Read the model definition and answer for the solid it produces. Units are mm, in the model's axes. A direction names the side the tool comes from. Coordinates: 2 decimals unless noted, no trailing zeros. Loops run counter-clockwise (first coordinate to the right, second up) from the corner with the lowest first, then second, coordinate; pieces in that order, holes last. Notation, with made-up numbers: (54, -11) - (86, -11) arc R7 cw to (86, -1) - close; hole circle Ø6 at (71.25, 7.25). An arc over 180 degrees is marked (long way). Use one line per item in the form item = value.
Autodesk Inventor part; units mm, degrees
ref_plane "YZ Plane" through (0, 0, 0) normal (1, 0, 0) x (0, 1, 0)
ref_plane "XZ Plane" through (0, 0, 0) normal (0, 1, 0) x (-1, 0, 0)
ref_plane "XY Plane" through (0, 0, 0) normal (0, 0, 1) x (1, 0, 0)
sketch "Sketch1" plane through (0, 0, 0) normal (0, 1, 0) x (-1, 0, 0)
  circle A0 centre (0, 12.75) radius 8.05
  circle A1 centre (0, -12.75) radius 8.05
  line L0 (14.5, 27) -> (-14.5, 27)
  line L1 (-14.5, 27) -> (-14.5, -27)
  line L2 (-14.5, -27) -> (14.5, -27)
  line L3 (14.5, -27) -> (14.5, 27)
  line L4 (14.5, 27) -> (-14.5, -27) construction
  line L5 (-14.5, 27) -> (14.5, -27) construction
  point P0 (0, 0)
  dimension "d0" = 16.1
  dimension "d1" = 16.1
  dimension "d2" = 25.5
  dimension "d3" = 29
  dimension "d4" = 54
  dimension "d5" = 14.5
  dimension "d6" = 14.5
  dimension "d7" = 14.25
  dimension "d8" = 14.25
extrude "Extrusion1" add sketch "Sketch1" along normal blind 3
sketch "Sketch2" plane through (0, 3, 0) normal (0, 1, 0) x (1, 0, 0)
  line L0 (-11.5, -24) -> (11.5, -24)
  line L1 (11.5, -24) -> (11.5, 24)
  line L2 (11.5, 24) -> (-11.5, 24)
  line L3 (-11.5, 24) -> (-11.5, -24)
  line L4 (-11.5, -24) -> (11.5, 24) construction
  line L5 (11.5, -24) -> (-11.5, 24) construction
  line L6 (14.5, -27) -> (14.5, 27)
  line L7 (-14.5, -27) -> (14.5, -27)
  line L8 (14.5, -27) -> (14.5, 27)
  line L9 (14.5, 27) -> (-14.5, 27)
  line L10 (-14.5, 27) -> (-14.5, -27)
  line L11 (-14.5, -27) -> (14.5, 27) construction
  line L12 (14.5, -27) -> (-14.5, 27) construction
  point P0 (0, 0)
  dimension "d11" = 23
  dimension "d12" = 48
extrude "Extrusion2" add sketch "Sketch2" along normal blind 25
sketch "Sketch3" plane through (0, 28, 0) normal (0, 1, 0) x (1, 0, 0)
  line L0 (-25.5, 27) -> (25.5, 27)
  line L1 (25.5, 27) -> (25.5, -27)
  line L2 (25.5, -27) -> (-25.5, -27)
  line L3 (-25.5, -27) -> (-25.5, 27)
  line L4 (-25.5, 27) -> (25.5, -27) construction
  line L5 (25.5, 27) -> (-25.5, -27) construction
  line L6 (14.5, -27) -> (14.5, 27)
  line L7 (-14.5, 27) -> (14.5, 27)
  line L8 (14.5, 27) -> (14.5, -27)
  line L9 (14.5, -27) -> (-14.5, -27)
  line L10 (-14.5, -27) -> (-14.5, 27)
  line L11 (-14.5, 27) -> (14.5, -27) construction
  line L12 (14.5, 27) -> (-14.5, -27) construction
  point P0 (0, 0)
  dimension "d15" = 51
extrude "Extrusion3" add sketch "Sketch3" against normal blind 3 contours L0 L10 L2 L3 | L0 L1 L2 L6
sketch "Sketch4" plane through (0, 28, 0) normal (0, 1, 0) x (1, 0, 0)
  line L0 (-25.5, -27) -> (25.5, -27)
  line L1 (-25.5, 27) -> (25.5, 27)
  line L2 (25.5, 27) -> (25.5, -27)
  line L3 (25.5, -27) -> (-25.5, -27)
  line L4 (-25.5, -27) -> (-25.5, 27)
  line L5 (-25.5, 27) -> (25.5, -27) construction
  line L6 (25.5, 27) -> (-25.5, -27) construction
  line L7 (-22.5, 24) -> (22.5, 24)
  line L8 (22.5, 24) -> (22.5, -24)
  line L9 (22.5, -24) -> (-22.5, -24)
  line L10 (-22.5, -24) -> (-22.5, 24)
  line L11 (-22.5, 24) -> (22.5, -24) construction
  line L12 (22.5, 24) -> (-22.5, -24) construction
  point P0 (0, 0)
  dimension "d18" = 45
  dimension "d19" = 48
extrude "Extrusion4" add sketch "Sketch4" along normal blind 15
sketch "Sketch5" plane through (0, 28, 0) normal (0, 1, 0) x (1, 0, 0)
  line L0 (-11.5, 24) -> (-22.5, 24)
  line L1 (-22.5, 24) -> (-22.5, -24)
  line L2 (-22.5, -24) -> (-11.5, -24)
  line L3 (-11.5, -24) -> (-11.5, 24)
  line L4 (22.5, 24) -> (11.5, 24)
  line L5 (11.5, 24) -> (11.5, -24)
  line L6 (11.5, -24) -> (22.5, -24)
  line L7 (22.5, -24) -> (22.5, 24)
  circle A0 centre (18.5, 20) radius 1.75
  line L8 (14.5, 27) -> (14.5, -27)
  line L9 (14.5, 27) -> (25.5, 27)
  line L10 (25.5, 27) -> (25.5, -27)
  line L11 (25.5, -27) -> (14.5, -27)
  line L12 (-11.5, 24) -> (-11.5, -24)
  line L13 (-11.5, -24) -> (11.5, -24)
  line L14 (11.5, -24) -> (11.5, 24)
  line L15 (11.5, 24) -> (-11.5, 24)
  circle A1 centre (0, 12.75) radius 8.05
  circle A2 centre (0, -12.75) radius 8.05
  circle A3 centre (18.5, -20) radius 1.75
  circle A4 centre (-18.5, 20) radius 1.75
  circle A5 centre (-18.5, -20) radius 1.75
  point P0 (0, 0)
  dimension "d22" = 3.5
  dimension "d23" = 4
  dimension "d24" = 4
  dimension "d25" = 4
  dimension "d28" = 40
  dimension "d31" = 37
  dimension "d53" = 4
extrude "Extrusion5" cut sketch "Sketch5" against normal blind 10 contours A0 | A3 | A4 | A5
chamfer "Chamfer1" distance 2 angle 45 4 edges at (-14.5, 0, 0) (14.5, 0, 0) (0, 0, 27) (0, 0, -27)
chamfer "Chamfer2" distance 2 angle 45 2 edges at (-14.5, 25, 0) (14.5, 25, 0)
sketch "Sketch6" plane through (0, 25, 0) normal (0, -1, 0) x (1, 0, 0)
  line L0 (-16.5, 27) -> (-16.5, -27)
  circle A0 centre (-18.5, -20) radius 1.75
  circle A1 centre (-18.5, 20) radius 1.75
  line L1 (-16.5, 27) -> (-25.5, 27)
  line L2 (-25.5, 27) -> (-25.5, -27)
  line L3 (-25.5, -27) -> (-16.5, -27)
  line L4 (16.5, -27) -> (16.5, 27)
  circle A2 centre (18.5, -20) radius 1.75
  line L5 (16.5, -27) -> (25.5, -27)
  line L6 (25.5, -27) -> (25.5, 27)
  line L7 (25.5, 27) -> (16.5, 27)
  circle A3 centre (18.5, 20) radius 1.75
  circle A4 centre (18.5, -20) radius 3
  circle A5 centre (18.5, 20) radius 3
  circle A6 centre (-18.5, -20) radius 3
  circle A7 centre (-18.5, 20) radius 3
  point P0 (0, 0)
  dimension "d42" = 6
  dimension "d45" = 40
  dimension "d48" = 37
extrude "Extrusion6" cut sketch "Sketch6" along normal blind 10 contours A7 L0 | L0 A7 | A6 L0 | L0 A6 | A0 | A1 | A4 L4 | L4 A4 | A5 L4 | L4 A5 | A2 | A3
sketch "Sketch7" plane through (25.5, 43, -27) normal (0, 0, -1) x (-1, 0, 0)
  line L0 (40, -41) -> (11, -41)
  line L1 (40, -41) -> (40, -20)
  line L2 (42, -18) -> (40, -20)
  line L3 (51, -18) -> (42, -18)
  line L4 (51, 0) -> (51, -18)
  line L5 (0, 0) -> (51, 0)
  line L6 (0, -18) -> (0, 0)
  line L7 (9, -18) -> (0, -18)
  line L8 (11, -20) -> (9, -18)
  line L9 (11, -41) -> (11, -20)
  line L10 (0, 0) -> (51, 0)
  line L11 (18, 0) -> (33, 0)
  line L12 (33, 0) -> (33, -3)
  line L13 (33, -3) -> (18, -3)
  line L14 (18, -3) -> (18, 0)
  point P0 (25.5, -43)
  dimension "d54" = 15
  dimension "d55" = 3
  dimension "d56" = 18
  dimension "d57" = 18
extrude "Extrusion7" add sketch "Sketch7" along normal blind 16 contours L12 L13 L14 L5
chamfer "Chamfer3" distance 2 angle 45 3 edges at (0, 40, -27) (-7.5, 41.5, -27) (7.5, 41.5, -27)
sketch "Sketch8" plane through (-7.5, 40, -43) normal (0, -1, 0) x (1, 0, 0)
  line L0 (0, 14) -> (15, 14)
  line L1 (0, 14) -> (0, 0)
  line L2 (15, 0) -> (0, 0)
  line L3 (15, 14) -> (15, 0)
  circle A0 centre (7.5, 7) radius 3
  point P0 (7.5, 43)
  dimension "d63" = 6
equation "\"d7\" = d8"
equation "\"d23\" = d24"
equation "\"d25\" = d53"
equation "\"d56\" = d57"
properties part number "obudowa_baza"
Item 1: The part is cut by section B-B on x = 18.5. Give the vertices of the cut face in (y, z).
Results below:
outline = (25, -27) - (43, -27) - (43, -24) - (28, -24) - (28, -21.75) - (25, -21.75) - close; (25, -18.25) - (28, -18.25) - (28, 18.25) - (25, 18.25) - close; (25, 21.75) - (28, 21.75) - (28, 24) - (43, 24) - (43, 27) - (25, 27) - close
Item 2: The part is cut by section D-D on y = 26. Give the vertices of the cut face in (x, z), plus the area to 3 significant figures.
Results below:
outline = (-25.5, -27) - (25.5, -27) - (25.5, 27) - (-25.5, 27) - close; hole circle Ø3.5 at (-18.5, -20); hole circle Ø3.5 at (-18.5, 20); hole (-11.5, -24) - (11.5, -24) - (11.5, 24) - (-11.5, 24) - close; hole circle Ø3.5 at (18.5, -20); hole circle Ø3.5 at (18.5, 20)
area = 1,610 mm²
Item 3: Find the intervals of material crossed by L1, parallel to Z at x = -18.5, y = 26.7; L2, parallel to Z at x = 3.5, y = 8.5; L3, parallel to X at y = 25.7, z = -20, in increasing order.
Results below:
L1 = -27 to -21.75, -18.25 to 18.25, 21.75 to 27
L2 = -27 to -24, 24 to 27
L3 = -25.5 to -20.25, -16.75 to -11.5, 11.5 to 16.75, 20.25 to 25.5
Item 4: Which of the six approach directions +Z, -Z, +X, -X, +Y, -Y give full straight-line access (tool end or side, diameter ignored) to faces 4 (the flat face through (0, 27, 24)), 5 (the cylindrical face through (-18.728, 26.521, -21.735)), 6 (the flat face through (0, 40, -36)), 7 (the flat face through (-7.5, 42, -36))?
Results below:
face_4 = +Y
face_5 = +Y, -Y
face_6 = -Z, +X, -X, -Y
face_7 = -Z, -X, +Y, -Y
Item 5: The part is cut by section C-C on y = 5.5. Give the vertices of the cut face in (x, z), plus the area to 3 significant figures.
Results below:
outline = (-14.5, -27) - (14.5, -27) - (14.5, 27) - (-14.5, 27) - close; hole (-11.5, -24) - (11.5, -24) - (11.5, 24) - (-11.5, 24) - close
area = 462 mm²
Item 6: For a pull along X with two mould halves and no side action, classify faces 1 (the flat face through (17, 28, 0)), 2 (the flat face through (0, 42, -43)), 3 (the flat face through (8.5, 41, -28)) as +X half, -X half, draft (parallel to the pull), parting line (faces both ways), or undercut.
Results below:
face_1 = undercut
face_2 = draft
face_3 = +X half
Item 7: The part is cut by section A-A on z = -12.75. Give the vertices of the cut face in (x, y).
Results below:
outline = (-25.5, 25) - (-16.5, 25) - (-14.5, 23) - (-14.5, 2) - (-12.5, 0) - (-8.05, 0) - (-8.05, 3) - (-11.5, 3) - (-11.5, 28) - (-22.5, 28) - (-22.5, 43) - (-25.5, 43) - close; (8.05, 0) - (12.5, 0) - (14.5, 2) - (14.5, 23) - (16.5, 25) - (25.5, 25) - (25.5, 43) - (22.5, 43) - (22.5, 28) - (11.5, 28) - (11.5, 3) - (8.05, 3) - close
Item 8: Each of these flat-tipped pins is pushed along its axis until it touches: P1, Ø17, axis at y = 15, z = 13, coming from the -X side; P2, Ø7, axis at x = -3, z = -34, coming from the -Y side; P3, Ø12, axis at y = 10.5, z = -16.5, coming from the +X side. Where does it stop, or does it pass through?
Results below:
P1 = -15
P2 = 40
P3 = 14.5
